Here's how the part is built. I have some questions about the finished solid (model axes, mm). Coordinates: 2 decimals unless noted, no trailing zeros. Use a Markdown table: item, result. Add a question column.
Item 1: If I drill on line 1 along Y through (x, z) = (-4.5, 0.85); line 2 along Y through (x, z) = (-44, 0.9); line 3 along X through (y, z) = (-20.5, 0.4), over which ranges is the centre line in solid material (lowest first)? Write a range as from..to.
Item 2: Will this pin go through, and if not, where does the flat tip stop? pin 1 Ø11 at (x, y) = (-173.785, -13.1) entering from +Z.
Item 3: Imagine slicing it at A-A, the plane z = 0.55. Count the separate pieces of the cut face and the enclosed holes in it, and give its area (3 significant figures).
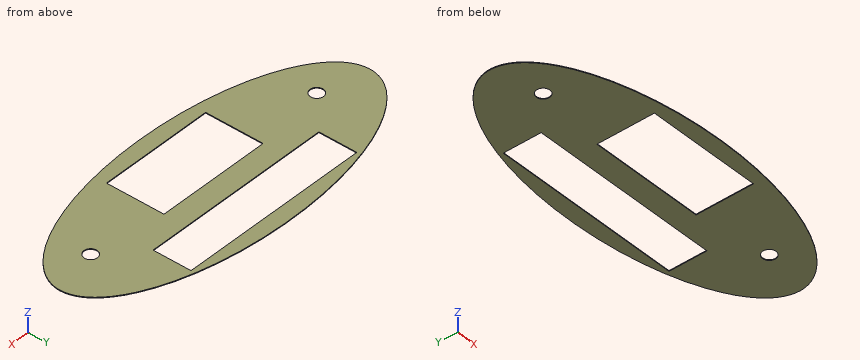
```python
from build123d import *

# Parameters (mm, degrees)
FUSELAGE_FRONT_RX          = 238.17677875
FUSELAGE_FRONT_RY          = 100
FUSELAGE_FRONT_R           = 9
FUSELAGE_FRONT_W           = 254.8
FUSELAGE_FRONT_H           = 50.8
FUSELAGE_FRONT_W_2         = 152.4
FUSELAGE_FRONT_H_2         = 77
FUSELAGE_FRONT_PLATE_DEPTH = 1


with BuildPart() as part:
    # fuselage_front → fuselage_front_plate (new body)
    with BuildSketch(Plane.XY):
        with Locations(Location((0, 1.9), (0, 0, 0))):
            Ellipse(FUSELAGE_FRONT_RX, FUSELAGE_FRONT_RY)
        with Locations((173.785, -13.1)):
            Circle(FUSELAGE_FRONT_R, mode=Mode.SUBTRACT)
        with Locations(Location((-173.785, -13.1, 0), (0, 0, 180))):
            Circle(FUSELAGE_FRONT_R, mode=Mode.SUBTRACT)
        with Locations((0, 55.4)):
            Rectangle(FUSELAGE_FRONT_W, FUSELAGE_FRONT_H, mode=Mode.SUBTRACT)
        with Locations((0, -38.5)):
            Rectangle(FUSELAGE_FRONT_W_2, FUSELAGE_FRONT_H_2, mode=Mode.SUBTRACT)
    extrude(amount=FUSELAGE_FRONT_PLATE_DEPTH)


solid = part.part
```
Ans:
| question | item | result |
|---|---|---|
| 1 | line 1 | y = -98.08..-77, 0..30, 80.8..101.88 |
| 1 | line 2 | y = -96.38..-77, 0..30, 80.8..100.18 |
| 1 | line 3 | x = -232.12..-178.91, -168.66..-76.2, 76.2..168.66, 178.91..232.12 |
| 2 | pin 1 | passes through |
| 3 | separate pieces | 1 |
| 3 | enclosed holes | 4 |
| 3 | area | 49,600 mm^2 |
